Check sheet for the modelled part. Datum: model origin and axes. Units: mm. A direction names the side the tool comes from. Coordinates: 2 decimals unless noted, no trailing zeros. Loops run counter-clockwise (first coordinate to the right, second up) from the corner with the lowest first, then second, coordinate; pieces in that order, holes last. Notation, with made-up numbers: (76.5, 70.5) -> (118.5, 70.5) arc R27 cw to (118.5, 91.5) -> close; hole circle Ø2 at (87.25, 75.25). An arc over 180 degrees is marked (long way). Use CSV: the item, a comma, the result in double quotes. Start each with the question number.
1. Gauge pin test, flat ends, axial feed: pin 1 (1.8 mm diameter, centred on x = 152.5, z = -134, fed in from +Y); pin 2 (1.8 mm diameter, centred on x = 57, y = 2.5, fed in from +Z); pin 3 (12 mm diameter, centred on x = 78, y = 14.5, fed in from +Z). Record the tip position at first contact, or that the pin passes through.
2. Sectioned sample at B-B, the plane x = 137. Record the cut outline in (y, z).
3. Release check for a two-part mould opening along X. For faces 4 (the face through (1.6, 14, -147)), 5 (the face through (0, 13, -148)), 6 (the face through (140, 1.6, -135)), 7 (the face through (153.2, 13, -148)) record: pulls with the +X half, pulls with the -X half, needs draft (parallel to the pull), parting line crosses it, or undercut.
4. Set-up check for faces 1 (the face through (151.6, 14, -147)), 2 (the face through (76, 1.6, -287)), 3 (the face through (13, 0, -148)): record each of +Z, -Z, +X, -X, +Y, -Y from which the full face is reachable in a straight line by a thin tool's end or side.
5. Sectioned sample at C-C, the plane y = 13.5. Record the cut outline in (x, z).
6. Thickness scan on L1, parallel to X at y = 4.25, z = -249; L2, parallel to Z at x = 120, y = 19; L3, parallel to Y at x = 13, z = -157.5. Record the ranges inside material, lowest first.
7. Sectioned sample at A-A, the plane z = -250. Record the cut outline in (x, y).
8. Sectioned sample at D-D, the plane x = 57.5. Record the cut outline in (y, z), and give its area (3 significant figures).
```python
from build123d import *

# Parameters (mm, degrees)
BOSS_EXTRUDE1_DEPTH   = 300
BOSS_EXTRUDE1_2_DEPTH = 300
BOSS_EXTRUDE2_DEPTH   = 150


with BuildPart() as part:
    # Sketch1 → Boss-Extrude1 (new body)
    with BuildSketch(Plane.XY):
        Polygon((25.4, 0), (0, 0), (0, 25.4), (1.6002, 25.4), (1.6002, 1.6002), (25.4, 1.6002), align=None)
    extrude(amount=-BOSS_EXTRUDE1_DEPTH)



with BuildPart() as body_2:
    # Sketch1 → Boss-Extrude1 2 (new body)
    with BuildSketch(Plane.XY):
        Polygon((153.2004, 25.4), (151.6002, 25.4), (151.6002, 1.6002), (127.8004, 1.6002), (127.8004, 0), (153.2004, 0), align=None)
    extrude(amount=-BOSS_EXTRUDE1_2_DEPTH)


with BuildPart() as part_1:
    add(part.part)

    add(body_2.part)  # Boss-Extrude2 merges body 2
    # Sketch2 → Boss-Extrude2 (add)
    with BuildSketch(Plane(origin=(1.6002, 0, 0), x_dir=(0, 0, -1), z_dir=(1, 0, 0))):
        Polygon((274.6, 1.6002), (300, 1.6002), (300, 27.0002), (298.3998, 27.0002), (298.3998, 3.2004), (274.6, 3.2004), align=None)
    extrude(amount=BOSS_EXTRUDE2_DEPTH)


solid = part_1.part
```
Completed:
1,pin 1,"y = 25.4"
1,pin 2,"z = -274.6"
1,pin 3,"z = -298.4"
2,outline,"(0, -300) -> (27, -300) -> (27, -298.4) -> (3.2, -298.4) -> (3.2, -274.6) -> (1.6, -274.6) -> (1.6, 0) -> (0, 0) -> close"
3,face 4,"undercut"
3,face 5,"pulls with the -X half"
3,face 6,"undercut"
3,face 7,"pulls with the +X half"
4,face 1,"+Z, +Y"
4,face 2,"+Z, -Z, -Y"
4,face 3,"+Z, -Z, +X, -X, -Y"
5,outline,"(0, -300) -> (153.2, -300) -> (153.2, 0) -> (151.6, 0) -> (151.6, -298.4) -> (1.6, -298.4) -> (1.6, 0) -> (0, 0) -> close"
6,L1,"0 to 1.6, 151.6 to 153.2"
6,L2,"-300 to -298.4"
6,L3,"0 to 1.6"
7,outline,"(0, 0) -> (25.4, 0) -> (25.4, 1.6) -> (1.6, 1.6) -> (1.6, 25.4) -> (0, 25.4) -> close; (127.8, 0) -> (153.2, 0) -> (153.2, 25.4) -> (151.6, 25.4) -> (151.6, 1.6) -> (127.8, 1.6) -> close"
8,outline,"(1.6, -300) -> (27, -300) -> (27, -298.4) -> (3.2, -298.4) -> (3.2, -274.6) -> (1.6, -274.6) -> close"
8,area,"78.7 mm²"
